The model under review builds one solid part; all positions refer to its coordinate system, in mm. A direction names the side the tool comes from. Round coordinates to 2 decimals unless told otherwise and drop trailing zeros. Loops run counter-clockwise (first coordinate to the right, second up) from the corner with the lowest first, then second, coordinate; pieces in that order, holes last. Notation, with made-up numbers: M 44,84.5 L 99,84.5 A19 ccw 99,112.5 Z; hole C 53,-23 d6. An arc over 180 degrees is marked long. One line per question, with ' | ' between items.
from build123d import *

# Parameters (mm, degrees)
MODEL_R                  = 8.05
MODEL_W                  = 25.8
MODEL_H                  = 11.3
SALIENTE_EXTRUIR1_DEPTH  = 3
CROQUIS2_W               = 38.3
CROQUIS2_H               = 12.1
CORTAR_EXTRUIR1_DEPTH    = 1
CROQUIS3_W               = 3
CROQUIS3_H               = 36.5
SALIENTE_EXTRUIR2_DEPTH  = 15.8
CROQUIS4_R               = 0.75
CROQUIS4_W               = 11.8
CROQUIS4_H               = 22.5
CORTAR_EXTRUIR2_DEPTH    = 3
CROQUIS5_R               = 1.5
CORTAR_EXTRUIR3_DEPTH    = 1
REDONDEO1_R              = 2
REDONDEO1_OF_SIMETR_A1_R = 2
REDONDEO2_R              = 2
CROQUIS6_W               = 20
CROQUIS6_H               = 3
SALIENTE_EXTRUIR3_DEPTH  = 8
CROQUIS7_R               = 1.5
CORTAR_EXTRUIR4_DEPTH    = 3
CROQUIS8_R               = 2.25
CORTAR_EXTRUIR5_DEPTH    = 1
REDONDEO3_R              = 2


with BuildPart() as part:
    # Model → Saliente-Extruir1 (new body)
    with BuildSketch(Plane.XY):
        with BuildLine():
            Line((102.870799912, -11.520997464), (102.870799912, -48.020997464))
            Line((102.870799912, -48.020997464), (96.870799912, -48.020997464))
            ThreePointArc((96.870799912, -48.020997464), (95.456586349, -48.606783901), (94.870799912, -50.020997464))
            Line((94.870799912, -50.020997464), (94.870799912, -51.020997464))
            ThreePointArc((94.870799912, -51.020997464), (94.285013474, -52.435211026), (92.870799912, -53.020997464))
            Line((92.870799912, -53.020997464), (72.589823504, -53.020997464))
            ThreePointArc((72.589823504, -53.020997464), (71.175609941, -53.606783901), (70.589823504, -55.020997464))
            Line((70.589823504, -55.020997464), (70.589823504, -56.021223523))
            Line((70.589823504, -56.021223523), (50.589823504, -56.021223523))
            Line((50.589823504, -56.021223523), (50.589823504, -55.021203031))
            ThreePointArc((50.589823504, -55.021203031), (50.004044311, -53.606996713), (48.589843996, -53.021203031))
            Line((48.589843996, -53.021203031), (28.527119253, -53.020997464))
            ThreePointArc((28.527119253, -53.020997464), (27.112905691, -52.435211026), (26.527119253, -51.020997464))
            Line((26.527119253, -51.020997464), (26.527119253, -50.020997464))
            ThreePointArc((26.527119253, -50.020997464), (25.941332816, -48.606783901), (24.527119253, -48.020997464))
            Line((24.527119253, -48.020997464), (18.527119253, -48.020997464))
            Line((18.527119253, -48.020997464), (18.527119253, -11.520997464))
            Line((18.527119253, -11.520997464), (24.527119253, -11.520997464))
            ThreePointArc((24.527119253, -11.520997464), (25.941332816, -10.935211026), (26.527119253, -9.520997464))
            Line((26.527119253, -9.520997464), (26.527119253, 4.938044993))
            ThreePointArc((26.527119253, 4.938044993), (30.595611796, 12.168478816), (38.618250464, 14.282497178))
            ThreePointArc((38.618250464, 14.282497178), (37.976525569, 11.63682094), (38.471226177, 8.959754465))
            ThreePointArc((38.471226177, 8.959754465), (43.800023098, 13.598439583), (50.438823204, 16.015009344))
            ThreePointArc((50.438823204, 16.015009344), (49.41482724, 13.510261305), (50.461877073, 11.015062492))
            ThreePointArc((50.461877073, 11.015062492), (55.039384462, 14.390193601), (60.387431279, 16.325000863))
            ThreePointArc((60.387431279, 16.325000863), (62.464845981, 11.626325475), (66.424253692, 8.352750544))
            ThreePointArc((66.424253692, 8.352750544), (73.028771683, 13.03256979), (80.697857855, 15.622064598))
            ThreePointArc((80.697857855, 15.622064598), (84.601159243, 8.674615803), (92.204558947, 6.289009084))
            ThreePointArc((92.204558947, 6.289009084), (92.573891536, 6.246895811), (92.902325099, 6.072793877))
            ThreePointArc((92.902325099, 6.072793877), (94.353114302, 4.250236817), (94.870799912, 1.979002536))
            Line((94.870799912, 1.979002536), (94.870799912, -9.520997464))
            ThreePointArc((94.870799912, -9.520997464), (95.456586349, -10.935211026), (96.870799912, -11.520997464))
            Line((96.870799912, -11.520997464), (102.870799912, -11.520997464))
        make_face()
        with Locations((73.589823504, -8.020694487)):
            Circle(MODEL_R, mode=Mode.SUBTRACT)
        with Locations((47.589823504, -8.020694487)):
            Circle(MODEL_R, mode=Mode.SUBTRACT)
        with Locations((60.589823504, -33.326919867)):
            Rectangle(MODEL_W, MODEL_H, mode=Mode.SUBTRACT)
    extrude(amount=SALIENTE_EXTRUIR1_DEPTH)

    # Croquis2 → Cortar-Extruir1 (cut)
    with BuildSketch(Plane(origin=(0, 0, 0), x_dir=(-1, 0, 0), z_dir=(0, 0, -1))):
        with Locations((-61.789823504, -33.326919867)):
            Rectangle(CROQUIS2_W, CROQUIS2_H)
    extrude(amount=-CORTAR_EXTRUIR1_DEPTH, mode=Mode.SUBTRACT)

    # Croquis3 → Saliente-Extruir2 (add)
    with BuildSketch(Plane(origin=(0, 0, 0), x_dir=(-1, 0, 0), z_dir=(0, 0, -1))):
        with Locations((-101.370799912, -29.770997464)):
            Rectangle(CROQUIS3_W, CROQUIS3_H)
    saliente_extruir2 = extrude(amount=SALIENTE_EXTRUIR2_DEPTH)

    # Croquis4 → Cortar-Extruir2 (cut)
    with BuildSketch(Plane(origin=(102.870799912, 0, 0), x_dir=(0, 0, -1), z_dir=(1, 0, 0))):
        with Locations((7.9, -43.420997464)):
            Circle(CROQUIS4_R)
        with Locations((7.9, -16.120997464)):
            Circle(CROQUIS4_R)
        with Locations((7.9, -29.770997464)):
            Rectangle(CROQUIS4_W, CROQUIS4_H)
    cortar_extruir2 = extrude(amount=-CORTAR_EXTRUIR2_DEPTH, mode=Mode.SUBTRACT)

    # Croquis5 → Cortar-Extruir3 (cut)
    with BuildSketch(Plane(origin=(102.870799912, 0, 0), x_dir=(0, 0, -1), z_dir=(1, 0, 0))):
        with Locations((7.9, -16.120997464)):
            Circle(CROQUIS5_R)
        with Locations((7.9, -43.420997464)):
            Circle(CROQUIS5_R)
    cortar_extruir3 = extrude(amount=-CORTAR_EXTRUIR3_DEPTH, mode=Mode.SUBTRACT)

    # Redondeo1
    redondeo1_edges = [part.edges().sort_by_distance(p)[0] for p in [
        (101.370799912, -48.020997464, -15.8),
        (101.370799912, -11.520997464, -15.8),
    ]]
    fillet(redondeo1_edges, radius=REDONDEO1_R)

    # Simetría1: Saliente-Extruir2, Cortar-Extruir2, Cortar-Extruir3 across plane
    add(saliente_extruir2.mirror(Plane(origin=(60.700799912, 0, 0), x_dir=(0, 0, 1), z_dir=(1, 0, 0))))
    add(cortar_extruir2.mirror(Plane(origin=(60.700799912, 0, 0), x_dir=(0, 0, 1), z_dir=(1, 0, 0))), mode=Mode.SUBTRACT)
    add(cortar_extruir3.mirror(Plane(origin=(60.700799912, 0, 0), x_dir=(0, 0, 1), z_dir=(1, 0, 0))), mode=Mode.SUBTRACT)

    # Redondeo1 of Simetría1
    redondeo1_of_simetr_a1_edges = [part.edges().sort_by_distance(p)[0] for p in [
        (20.030799912, -48.020997464, -15.8),
        (20.030799912, -11.520997464, -15.8),
    ]]
    fillet(redondeo1_of_simetr_a1_edges, radius=REDONDEO1_OF_SIMETR_A1_R)

    # Redondeo2
    redondeo2_edges = [part.edges().sort_by_distance(p)[0] for p in [
        (18.527119253, -29.770997464, 3),
        (102.870799912, -29.770997464, 3),
    ]]
    fillet(redondeo2_edges, radius=REDONDEO2_R)

    # Croquis6 → Saliente-Extruir3 (add)
    with BuildSketch(Plane(origin=(0, 0, 0), x_dir=(-1, 0, 0), z_dir=(0, 0, -1))):
        with Locations((-60.589823504, -54.521223523)):
            Rectangle(CROQUIS6_W, CROQUIS6_H)
    extrude(amount=SALIENTE_EXTRUIR3_DEPTH)

    # Croquis7 → Cortar-Extruir4 (cut)
    with BuildSketch(Plane(origin=(0, -53.021223523, 0), x_dir=(1, 0, 0), z_dir=(0, 1, 0))):
        with Locations((66.589823504, 3.5)):
            Circle(CROQUIS7_R)
        with Locations((54.589823504, 3.5)):
            Circle(CROQUIS7_R)
    extrude(amount=-CORTAR_EXTRUIR4_DEPTH, mode=Mode.SUBTRACT)

    # Croquis8 → Cortar-Extruir5 (cut)
    with BuildSketch(Plane(origin=(0, -53.021223523, 0), x_dir=(1, 0, 0), z_dir=(0, 1, 0))):
        with Locations((66.589823504, 3.5)):
            Circle(CROQUIS8_R)
        with Locations((54.589823504, 3.5)):
            Circle(CROQUIS8_R)
    extrude(amount=-CORTAR_EXTRUIR5_DEPTH, mode=Mode.SUBTRACT)

    # Redondeo3
    redondeo3_edges = [part.edges().sort_by_distance(p)[0] for p in [
        (70.589823504, -54.521223523, -8),
        (50.589823504, -54.521223523, -8),
    ]]
    fillet(redondeo3_edges, radius=REDONDEO3_R)


solid = part.part
1) Machinability: for faces 5 (the flat face through (61, -53.021, -4)), 6 (the cylindrical face through (62.421, 11.684, 1.479)), 7 (the flat face through (101, -48.021, -5)), 8 (the cylindrical face through (19, -42.4, -6.8)), which of the approach directions +Z, -Z, +X, -X, +Y, -Y give a long, thin tool a straight path to every point of the face, cutting with its end or side? Answer none if there is none.
Output values:
face 5: -Z, +X, -X, +Y | face 6: +Z, -Z, +Y | face 7: +Z, -Z, +X, -Y | face 8: -X
2) Mouldability with a two-part tool opening along Y and no side actions: class faces 1 (the flat face through (101.871, -16, -7)), 2 (the cylindrical face through (25.926, -10.951, 1.479)), 3 (the cylindrical face through (81.026, -11.104, 1.479)), 4 (the cylindrical face through (27.13, -52.45, 1.48)) as +Y half, -Y half, draft (parallel to the pull), parting line (faces both ways), or undercut.
Output values:
face 1: undercut | face 2: +Y half | face 3: undercut | face 4: -Y half
3) Add section A-A on y = -3. State the section outline as (x, z) points.
Output values:
outline: M 26.53,0 L 41.3,0 L 41.3,3 L 26.53,3 Z; M 53.88,0 L 67.3,0 L 67.3,3 L 53.88,3 Z; M 79.88,0 L 94.87,0 L 94.87,3 L 79.88,3 Z
4) For line 1 (X direction, y = -53.3, z = -3.5); line 2 (Y direction, x = 18.8, z = -7.9); line 3 (Y direction, x = 20.6, z = -7.9), list the stretches that pass through material, from the lowest coordinate up.
Output values:
line 1: x = 50.59 to 52.34, 56.84 to 64.34, 68.84 to 70.59 | line 2: y = -48.02 to -44.92, -41.92 to -41.02, -18.52 to -17.62, -14.62 to -11.52 | line 3: y = -48.02 to -44.17, -42.67 to -41.02, -18.52 to -16.87, -15.37 to -11.52
5) Insertion check: P1, Ø1.5, axis at y = -55, z = 0.5, coming from the +X side; P2, Ø2.5, axis at x = 54.59, z = -3.5, coming from the -Y side; P3, Ø10, axis at x = 65, y = -5, coming from the -Z side; P4, Ø1.5, axis at y = -16, z = -8, coming from the +X side. Each pin has a flat end and moves straight along its axis. Give the tip position at first contact, or say it passes through.
Output values:
P1: stops at x = 70.74 | P2: passes through | P3: stops at z = 0 | P4: stops at x = 101.87
6) Add section B-B on y = 12.5. State the section outline as (x, z) points.
Output values:
outline: M 31.05,0 L 38.06,0 L 38.06,3 L 31.05,3 Z; M 42.14,0 L 49.57,0 L 49.57,3 L 42.14,3 Z; M 52.15,0 L 61.87,0 L 61.87,3 L 52.15,3 Z; M 72.03,0 L 81.61,0 L 81.61,3 L 72.03,3 Z
7) Add section C-C on z = -3.5. State how many separate pieces and enclosed holes the cut face has, then the cut area to 3 significant figures.
Output values:
separate pieces: 7 | enclosed holes: 0 | area: 123 mm²
